Autodesk Inventor part; units mm, degrees
ref_plane "YZ Plane" through (0, 0, 0) normal (1, 0, 0) x (0, 1, 0)
ref_plane "XZ Plane" through (0, 0, 0) normal (0, 1, 0) x (-1, 0, 0)
ref_plane "XY Plane" through (0, 0, 0) normal (0, 0, 1) x (1, 0, 0)
sketch "Skizze1" plane through (0, 0, 0) normal (0, 0, 1) x (1, 0, 0)
  line L0 (0, 30) -> (49, 30)
  line L1 (49, 30) -> (49, 0)
  line L2 (49, 0) -> (0, 0)
  line L3 (0, 0) -> (0, 30)
  line L4 (-9.8, 0) -> (58.8, 0)
  line L5 (0, -6) -> (0, 36)
  point P0 (0, 0)
  dimension "d0" = 49
  dimension "d1" = 30
extrude "Extrusion1" add sketch "Skizze1" along normal blind 1
sketch "Skizze2" plane through (0, 0, 0) normal (0, 0, -1) x (-1, 0, 0)
  circle A0 centre (-24.5, 16) radius 3.25
  line L0 (-49, 30) -> (0, 30)
  line L1 (0, 0) -> (-49, 0)
  circle A1 centre (-24.5, 16) radius 5.25
  line L2 (-41, 30) -> (-8, 30)
  line L3 (-8, 30) -> (-8, 2)
  line L4 (-8, 2) -> (-41, 2)
  line L5 (-41, 2) -> (-41, 30)
  line L6 (-49, 0) -> (-49, 30)
  line L7 (0, 30) -> (0, 0)
  line L8 (-24.5, 30) -> (-24.5, 2)
  dimension "d4" = 6.5
  dimension "d5" = 10.5
  dimension "d8" = 2
  dimension "d9" = 8
  dimension "d10" = 8
  dimension "d11" = 14
extrude "Extrusion2" add sketch "Skizze2" along normal blind 6 contours A0 L8 A1 | A0 L8 A1
sketch "Skizze6" plane through (24.5, 16, 0) normal (0, 0, -1) x (-1, 0, 0)
  circle A0 centre (0, 0) radius 3.25
  circle A1 centre (0, 0) radius 3.25
  point P0 (24.5, -16)
extrude "Extrusion3" cut sketch "Skizze6" against normal through all
sketch "Skizze7" plane through (0, 0, 1) normal (0, 0, 1) x (1, 0, 0)
  line L0 (0, 30) -> (0, 0)
  line L1 (49, 30) -> (0, 30)
  point P0 (4, 26)
  point P1 (45, 26)
  point P2 (4, 4)
  point P3 (45, 4)
  dimension "d15" = 4
  dimension "d16" = 4
  dimension "d19" = 41
  dimension "d22" = 22
hole "Bohrung1" at (4, 26, 1) at (45, 26, 1) at (4, 4, 1) at (45, 4, 1) direction (0, 0, -1) diameter 4 end through all
properties part number "RE-Halter"
Read the model definition and answer for the solid it produces. Units are mm, in the model's axes. A direction names the side the tool comes from. Round coordinates to 2 decimals unless told otherwise and drop trailing zeros. Write each loop counter-clockwise with the first axis right and the second up, starting at its lowest first coordinate (ties: lowest second). Pieces come first, ordered by that corner, then holes.
Q1. Find section D-D on z = -0.5. Determine the outline of the cut face in (x, y), and give its area (3 significant figures).
Values:
outline: circle Ø10.5 at (24.5, 16); hole circle Ø6.5 at (24.5, 16)
area: 53.4 mm2
Q2. The mould has two halves that part along Y. Classify faces 3 (the face through (46.952, 26.434, 0.493)), 4 (the face through (26.895, 18.197, -2.549)), 5 (the face through (0, 14.8, 0.5)), 6 (the face through (24.2, 30, 0.5)): released by +Y, released by -Y, zero draft, split by the parting line, or undercut.
Values:
face 3: undercut
face 4: undercut
face 5: zero draft
face 6: released by +Y
Q3. A tool of negligible diameter and unlimited length cuts with its end or side. For faces 1 (the face through (49, 15.2, 0.5)), 2 (the face through (28.37, 12.45, -2.96)), from which of +Z, -Z, +X, -X, +Y, -Y can it reach the whole face along a straight path? Write none if from no direction.
Values:
face 1: +Z, -Z, +X, +Y, -Y
face 2: -Z
Q4. Find section A-A on x = 45. Determine the outline of the cut face in (y, z).
Values:
outline: (0, 0) - (2, 0) - (2, 1) - (0, 1) - close; (6, 0) - (24, 0) - (24, 1) - (6, 1) - close; (28, 0) - (30, 0) - (30, 1) - (28, 1) - close
Q5. Find section C-C on y = 22.25. Determine the outline of the cut face in (x, z), and give its area (3 significant figures).
Values:
outline: (0, 0) - (49, 0) - (49, 1) - (0, 1) - close
area: 49.0 mm2
Q6. Straight lines are drawn through the part: line 1 (X direction, y = 26, z = 0.4); line 2 (Y direction, x = 45, z = 0.5); line 3 (Y direction, x = 24.5, z = -0.5). For each, find the intervals that lie inside material, in ascending order.
Values:
line 1: x = 0 to 2, 6 to 43, 47 to 49
line 2: y = 0 to 2, 6 to 24, 28 to 30
line 3: y = 10.75 to 12.75, 19.25 to 21.25
Q7. Find section B-B on y = 26. Determine the outline of the cut face in (x, z).
Values:
outline: (0, 0) - (2, 0) - (2, 1) - (0, 1) - close; (6, 0) - (43, 0) - (43, 1) - (6, 1) - close; (47, 0) - (49, 0) - (49, 1) - (47, 1) - close
Q8. Flat-ended cylindrical pins translate along their axes: P1, Ø1, axis at x = 19.5, y = 12.5, coming from the -Z side; P2, Ø2, axis at y = 16, z = -4.5, coming from the -X side. Find the tip coordinate at first contact, or state that the pin passes through.
Values:
P1: stops at z = 0
P2: stops at x = 19.25
